Geometry: final body of the model. Coordinates: model frame, mm. Round coordinates to 2 decimals unless told otherwise and drop trailing zeros. Write each loop counter-clockwise with the first axis right and the second up, starting at its lowest first coordinate (ties: lowest second). Pieces come first, ordered by that corner, then holes.
from build123d import *

# Parameters (mm, degrees)
F1_DEPTH = 3


with BuildPart() as f1:
    # F0 (on Top) → F1 (new body)
    with BuildSketch(Plane.XY):
        with BuildLine():
            ThreePointArc((12.5, 4), (8.5, 0), (12.5, -4))
            Line((12.5, -4), (12.5, -2))
            ThreePointArc((12.5, -2), (10.5, 0), (12.5, 2))
            Line((12.5, 2), (12.5, 4))
        make_face()
        with BuildLine():
            Line((-12.5, -4), (12.5, -4))
            ThreePointArc((12.5, -4), (8.5, 0), (12.5, 4))
            Line((12.5, 4), (-12.5, 4))
            ThreePointArc((-12.5, 4), (-9.6715728753, 2.8284271247), (-8.5, 0))
            ThreePointArc((-8.5, 0), (-9.6715728753, -2.8284271247), (-12.5, -4))
        make_face()
        with BuildLine():
            Line((12.5, -2), (12.5, -4))
            ThreePointArc((12.5, -4), (15.3284271247, -2.8284271247), (16.5, 0))
            ThreePointArc((16.5, 0), (15.3284271247, 2.8284271247), (12.5, 4))
            Line((12.5, 4), (12.5, 2))
            ThreePointArc((12.5, 2), (13.9142135624, 1.4142135624), (14.5, 0))
            ThreePointArc((14.5, 0), (13.9142135624, -1.4142135624), (12.5, -2))
        make_face()
        with BuildLine():
            ThreePointArc((-12.5, 4), (-16.5, 0), (-12.5, -4))
            Line((-12.5, -4), (-12.5, -2))
            ThreePointArc((-12.5, -2), (-14.5, 0), (-12.5, 2))
            Line((-12.5, 2), (-12.5, 4))
        make_face()
        with BuildLine():
            Line((-12.5, -2), (-12.5, -4))
            ThreePointArc((-12.5, -4), (-9.6715728753, -2.8284271247), (-8.5, 0))
            ThreePointArc((-8.5, 0), (-9.6715728753, 2.8284271247), (-12.5, 4))
            Line((-12.5, 4), (-12.5, 2))
            ThreePointArc((-12.5, 2), (-11.0857864376, 1.4142135624), (-10.5, 0))
            ThreePointArc((-10.5, 0), (-11.0857864376, -1.4142135624), (-12.5, -2))
        make_face()
    extrude(amount=F1_DEPTH)


solid = f1.part
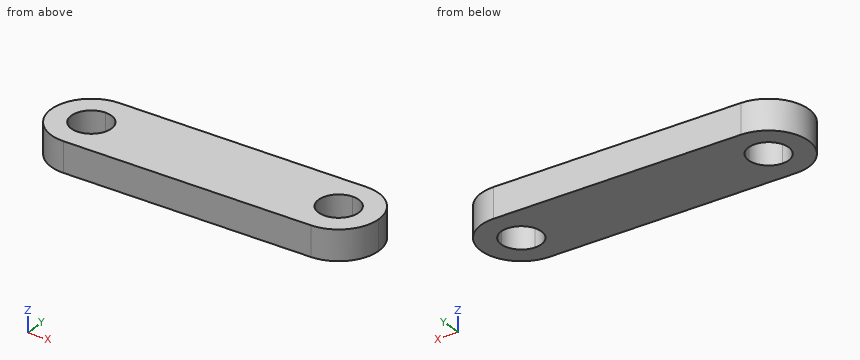
1) Section A-A on z = 1.9. Output: boundary loops of the cut face in (x, y), plus the area to 3 significant figures.
2) Section C-C on x = 13. Output: boundary loops of the cut face in (y, z), plus the area to 3 significant figures.
3) Line query: probe 1 along X at (y, z) = (-0.5, 0.35); probe 2 along X at (y, z) = (0.75, 2); probe 3 along Y at (x, z) = (12.5, 1.95). Output: solid intervals per line, ascending.
4) Section B-B on y = -0.75. Output: boundary loops of the cut face in (x, z), plus the area to 3 significant figures.
Filled in:
1. outline: (-12.5, -4) - (12.5, -4) arc R4 ccw to (12.5, 4) - (-12.5, 4) arc R4 ccw to start; hole circle Ø4 at (-12.5, 0); hole circle Ø4 at (12.5, 0)
1. area: 225 mm2
2. outline: (-3.97, 0) - (-1.94, 0) - (-1.94, 3) - (-3.97, 3) - close; (1.94, 0) - (3.97, 0) - (3.97, 3) - (1.94, 3) - close
2. area: 12.2 mm2
3. probe 1: x = -16.47 to -14.44, -10.56 to 10.56, 14.44 to 16.47
3. probe 2: x = -16.43 to -14.35, -10.65 to 10.65, 14.35 to 16.43
3. probe 3: y = -4 to -2, 2 to 4
4. outline: (-16.43, 0) - (-14.35, 0) - (-14.35, 3) - (-16.43, 3) - close; (-10.65, 0) - (10.65, 0) - (10.65, 3) - (-10.65, 3) - close; (14.35, 0) - (16.43, 0) - (16.43, 3) - (14.35, 3) - close
4. area: 76.3 mm2
